Autodesk Inventor part; units mm, degrees
ref_plane "YZ Plane" through (0, 0, 0) normal (1, 0, 0) x (0, 1, 0)
ref_plane "XZ Plane" through (0, 0, 0) normal (0, 1, 0) x (-1, 0, 0)
ref_plane "XY Plane" through (0, 0, 0) normal (0, 0, 1) x (1, 0, 0)
sketch "Sketch1" plane through (0, 0, 0) normal (0, 0, 1) x (1, 0, 0)
  line L0 (0, 0) -> (50.8, 0) construction
  line L1 (50.8, 0) -> (50.8, 50.3682) construction
  line L2 (50.8, 50.3682) -> (0, 50.3682) construction
  line L3 (0, 50.3682) -> (0, 0) construction
  circle A0 centre (50.8, 25.1841) radius 25.1841 construction
  line L4 (0, 0) -> (50.8, 0)
  line L5 (50.8, 0) -> (50.8, 50.3682) construction
  line L6 (50.8, 50.3682) -> (0, 50.3682)
  line L7 (0, 50.3682) -> (0, 0)
  arc A1 (50.8, 0) -> (50.8, 50.3682) centre (50.8, 25.1841) ccw
  dimension "d0" = 50.8
  dimension "d1" = 50.3682
extrude "Extrusion1" add sketch "Sketch1" along normal blind 3.175
sketch "Sketch2" plane through (0, 0, 3.175) normal (0, 0, 1) x (1, 0, 0)
  arc A0 (50.8, 0) -> (50.8, 50.3682) centre (50.8, 25.1841) ccw
  arc A1 (57.1075, 4.0982) -> (50.8, 47.1932) centre (50.8, 25.1841) ccw
  line L0 (27.3812, 15.6959) -> (33.7312, 15.6959)
  line L1 (33.7312, 15.6959) -> (33.7312, 34.7459)
  line L2 (33.7312, 34.7459) -> (27.3812, 34.7459)
  line L3 (27.3812, 34.7459) -> (27.3812, 15.6959)
  line L4 (27.3812, 15.6959) -> (33.7312, 34.7459) construction
  line L5 (33.7312, 15.6959) -> (27.3812, 34.7459) construction
  arc A2 (50.8, 47.1932) -> (30.9765, 34.7459) centre (50.8, 25.1841) ccw
  arc A3 (30.9411, 15.6959) -> (57.1075, 4.0982) centre (50.8, 25.1841) ccw
  line L6 (0, 50.3682) -> (0, 0)
  line L7 (50.8, 50.3682) -> (0, 50.3682)
  point P0 (30.5562, 25.2209)
  dimension "d6" = 3.175
  dimension "d7" = 6.35
  dimension "d8" = 19.05
  dimension "d9" = 12.4473
  dimension "d10" = 27.3812
  dimension "d11" = 15.6223
extrude "Extrusion2" cut sketch "Sketch2" against normal blind 3.175
sketch "Sketch3" plane through (0, 0, 3.175) normal (0, 0, 1) x (1, 0, 0)
  circle A0 centre (71.755, 25.1433) radius 1.1913
  line L0 (30.9411, 15.6959) -> (27.3812, 15.6959)
  line L1 (27.3812, 15.6959) -> (27.3812, 34.7459)
  line L2 (27.3812, 34.7459) -> (30.9765, 34.7459)
  arc A1 (30.9411, 15.6959) -> (30.9765, 34.7459) centre (50.8, 25.1841) ccw
  arc A2 (50.8, 0) -> (50.8, 50.3682) centre (50.8, 25.1841) ccw
  line L3 (50.8, 50.3682) -> (0, 50.3682)
  line L4 (0, 50.3682) -> (0, 0)
  line L5 (0, 0) -> (50.8, 0)
  point P0 (72.8091, 25.1433)
  point P1 (72.8006, 24.5725)
  point P2 (72.8028, 25.71)
  dimension "d14" = 2.3825
  dimension "d15" = 20.955
extrude "Extrusion3" add sketch "Sketch3" against normal up to surface (3.175 mm away) contours A1 A0 picked at (72.0601, 25.1427)
fillet "Fillet1" radius 3.302 2 edges at (72.8006, 24.5725, 1.5875) (72.8028, 25.71, 1.5875)
sketch "Sketch4" plane through (0, 0, 3.175) normal (0, 0, 1) x (1, 0, 0)
  line L0 (24.2062, 34.7459) -> (20.6502, 34.7459)
  line L1 (20.6502, 34.7459) -> (20.6502, 15.6959)
  line L2 (20.6502, 15.6959) -> (24.2062, 15.6959)
  line L3 (24.2062, 15.6959) -> (24.2062, 34.7459)
  line L4 (24.2062, 34.7459) -> (20.6502, 15.6959) construction
  line L5 (20.6502, 34.7459) -> (24.2062, 15.6959) construction
  line L6 (15.6502, 34.7459) -> (12.0942, 34.7459)
  line L7 (12.0942, 34.7459) -> (12.0942, 15.6959)
  line L8 (12.0942, 15.6959) -> (15.6502, 15.6959)
  line L9 (15.6502, 15.6959) -> (15.6502, 34.7459)
  line L10 (15.6502, 34.7459) -> (12.0942, 15.6959) construction
  line L11 (12.0942, 34.7459) -> (15.6502, 15.6959) construction
  line L12 (7.0942, 34.7459) -> (3.5382, 34.7459)
  line L13 (3.5382, 34.7459) -> (3.5382, 15.6959)
  line L14 (3.5382, 15.6959) -> (7.0942, 15.6959)
  line L15 (7.0942, 15.6959) -> (7.0942, 34.7459)
  line L16 (7.0942, 34.7459) -> (3.5382, 15.6959) construction
  line L17 (3.5382, 34.7459) -> (7.0942, 15.6959) construction
  line L18 (27.3812, 15.6959) -> (27.3812, 34.7459)
  line L19 (0, 50.3682) -> (0, 0)
  line L20 (27.3812, 34.7459) -> (30.9765, 34.7459)
  line L21 (27.9527, 9.9682) -> (10.1473, 9.9682) construction
  line L22 (25.4, 12.5209) -> (12.7, 12.5209)
  line L23 (12.7, 7.4155) -> (25.4, 7.4155)
  arc A0 (25.4, 7.4155) -> (25.4, 12.5209) centre (25.4, 9.9682) ccw
  arc A1 (12.7, 12.5209) -> (12.7, 7.4155) centre (12.7, 9.9682) ccw
  line L24 (27.9527, 40.4736) -> (10.1473, 40.4736) construction
  line L25 (25.4, 43.0263) -> (12.7, 43.0263)
  line L26 (12.7, 37.9209) -> (25.4, 37.9209)
  arc A2 (25.4, 37.9209) -> (25.4, 43.0263) centre (25.4, 40.4736) ccw
  arc A3 (12.7, 43.0263) -> (12.7, 37.9209) centre (12.7, 40.4736) ccw
  line L27 (30.9411, 15.6959) -> (27.3812, 15.6959)
  point P0 (22.4282, 25.2209)
  point P1 (13.8722, 25.2209)
  point P2 (5.3162, 25.2209)
  point P3 (27.3812, 25.2209)
  point P4 (19.05, 9.9682)
  point P5 (19.05, 40.4736)
  point P6 (27.9527, 40.4736)
  point P7 (12.0942, 25.2209)
  dimension "d19" = 3.175
  dimension "d20" = 5
  dimension "d21" = 5
  dimension "d22" = 3.556
  dimension "d23" = 3.556
  dimension "d24" = 3.556
  dimension "d25" = 19.05
  dimension "d26" = 19.05
  dimension "d27" = 19.05
  dimension "d28" = 3.5382
  dimension "d29" = 5.1054
  dimension "d30" = 5.1054
  dimension "d33" = 12.7
  dimension "d34" = 12.7
  dimension "d35" = 3.175
  dimension "d36" = 3.175
  dimension "d37" = 19.05
extrude "Extrusion4" cut sketch "Sketch4" against normal blind 25.4
fillet "Fillet2" radius 1.524 16 edges at (3.5382, 34.7459, 1.5875) (7.0942, 34.7459, 1.5875) (3.5382, 15.6959, 1.5875) (7.0942, 15.6959, 1.5875) (12.0942, 34.7459, 1.5875) (15.6502, 34.7459, 1.5875) (15.6502, 15.6959, 1.5875) (12.0942, 15.6959, 1.5875) (24.2062, 34.7459, 1.5875) (20.6502, 34.7459, 1.5875) (20.6502, 15.6959, 1.5875) (24.2062, 15.6959, 1.5875) (27.3812, 34.7459, 1.5875) (27.3812, 15.6959, 1.5875) (30.9411, 15.6959, 1.5875) (30.9765, 34.7459, 1.5875)
equation "\"d22\" = d23"
equation "\"d24\" = d23"
equation "\"d26\" = d25"
equation "\"d27\" = d25"
equation "\"d34\" = d33"
equation "\"d36\" = d35"
properties part number "EL2-009" material "Aluminum 6061"
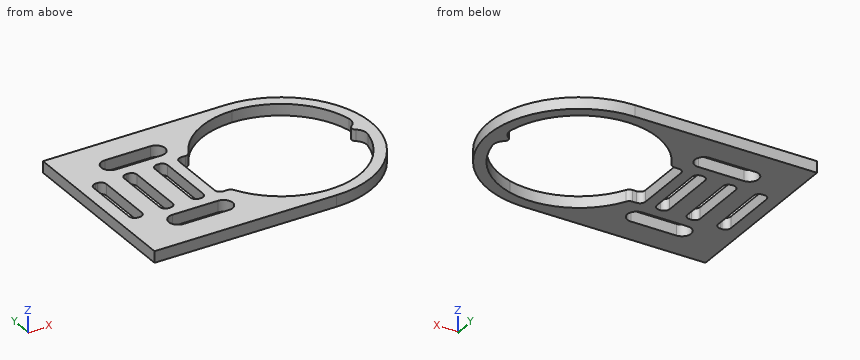
Read the model definition and answer for the solid it produces. Units are mm, in the model's axes. Coordinates: 2 decimals unless noted, no trailing zeros. Write each loop counter-clockwise with the first axis right and the second up, starting at its lowest first coordinate (ties: lowest second). Pieces come first, ordered by that corner, then holes. Notation, with made-up numbers: (61, -34.5) - (115, -34.5) arc R12 cw to (115, -30.5) - close; hole circle Ø3 at (-18, -20.5). An arc over 180 degrees is marked (long way). Answer as a JSON object with one key per item and string values. Group by question number.
1. This flat-tipped pin is pushed along its axis until it touches: P1, Ø1.6, axis at y = 28, z = 2, coming from the +X side. Where does it stop, or does it pass through?
2. A cutting plane is placed at D-D (z = 0.6). Give the number of separate pieces and of enclosed holes in the cut face, plus the area to 3 significant figures.
3. A cutting plane is placed at A-A (x = 43). Determine the outline of the cut face in (y, z) (3 decimals), plus the area to 3 significant figures.
4. A cutting plane is placed at B-B (y = 39). Determine the outline of the cut face in (x, z) (3 decimals), plus the area to 3 significant figures.
5. A cutting plane is placed at C-C (y = 18.5). Determine the outline of the cut face in (x, z) (3 decimals).
6. Consider L1, parallel to Y at x = 18.5, z = 2.8; L2, parallel to X at y = 25, z = 2.2; L3, parallel to X at y = 8, z = 2.9. Determine where each line is inside the solid, lowest interval first. Write a range as [from, to].
Worked out:
{
 "1": {"P1": "stops at x = 75.9"},
 "2": {"separate pieces": "1", "enclosed holes": "6", "area": "1,630 mm²"},
 "3": {"outline": "(0, 0) - (4.603, 0) - (4.603, 3.175) - (0, 3.175) - close; (45.765, 0) - (50.368, 0) - (50.368, 3.175) - (45.765, 3.175) - close", "area": "29.2 mm²"},
 "4": {"outline": "(0, 0) - (10.616, 0) - (10.616, 3.175) - (0, 3.175) - close; (27.484, 0) - (33.668, 0) - (33.668, 3.175) - (27.484, 3.175) - close; (67.932, 0) - (71.856, 0) - (71.856, 3.175) - (67.932, 3.175) - close", "area": "65.8 mm²"},
 "5": {"outline": "(0, 0) - (3.538, 0) - (3.538, 3.175) - (0, 3.175) - close; (7.094, 0) - (12.094, 0) - (12.094, 3.175) - (7.094, 3.175) - close; (15.65, 0) - (20.65, 0) - (20.65, 3.175) - (15.65, 3.175) - close; (24.206, 0) - (27.381, 0) - (27.381, 3.175) - (24.206, 3.175) - close; (71.77, 0) - (75.081, 0) - (75.081, 3.175) - (71.77, 3.175) - close"},
 "6": {"L1": "y = [0, 7.42], [12.52, 37.92], [43.03, 50.37]", "L2": "x = [0, 3.54], [7.09, 12.09], [15.65, 20.65], [24.21, 27.38], [70.57, 75.98]", "L3": "x = [0, 11.07], [27.03, 37.05], [64.55, 69.21]"}
}
